Autodesk Inventor part; units mm, degrees
ref_plane "YZ Plane" through (0, 0, 0) normal (1, 0, 0) x (0, 1, 0)
ref_plane "XZ Plane" through (0, 0, 0) normal (0, 1, 0) x (-1, 0, 0)
ref_plane "XY Plane" through (0, 0, 0) normal (0, 0, 1) x (1, 0, 0)
sketch "Sketch1" plane through (0, 0, 0) normal (1, 0, 0) x (0, 1, 0)
  circle A0 centre (0, 0) radius 7.9375
  dimension "d0" = 15.875
extrude "Extrusion1" add sketch "Sketch1" along normal blind 1.016
sketch "Sketch2" plane through (1.016, 0, 0) normal (1, 0, 0) x (0, 0, -1)
  point P0 (0, 0)
  point P1 (0, 0)
hole "Hole1" at (1.016, 0, 0) direction (-1, 0, 0) diameter 5.1054 end through all
fillet "Fillet1" radius 0.254 1 edges at (1.016, -7.9375, 0)
properties part number "PURCHASED,WASHER" material "Steel, Alloy"
Source: CAD feature listing. Evaluate the final solid. Frame: model axes, mm. Round coordinates to 2 decimals unless told otherwise and drop trailing zeros. Loops run counter-clockwise (first coordinate to the right, second up) from the corner with the lowest first, then second, coordinate; pieces in that order, holes last. Notation, with made-up numbers: M 68.5,84.25 L 103.5,84.25 A14 ccw 103.5,109.25 Z; hole C 70.5,4.5 d3. An arc over 180 degrees is marked long. Return JSON: item names as keys, results as strings. Group by question number.
1. Section query C-C on x = 0.35. Output: boundary loops of the cut face in (y, z) (1 decimal), and give its area (3 significant figures).
2. Section query A-A on z = 0. Output: boundary loops of the cut face in (x, y).
3. Material intervals for line 1 along Z through (x, y) = (0.55, 0); line 2 along Y through (x, z) = (0.5, 2.25), sorted ascending. Write a range as from..to.
Checks:
{
 "1": {"outline": "C 0,0 d15.9; hole C 0,0 d5.1", "area": "177 mm²"},
 "2": {"outline": "M 0,-7.94 L 0.76,-7.94 A0.25 ccw 1.02,-7.68 L 1.02,-2.55 L 0,-2.55 Z; M 0,2.55 L 1.02,2.55 L 1.02,7.68 A0.25 ccw 0.76,7.94 L 0,7.94 Z"},
 "3": {"line 1": "z = -7.94..-2.55, 2.55..7.94", "line 2": "y = -7.61..-1.21, 1.21..7.61"}
}
